from build123d import *

# Parameters (mm, degrees)
F1_DEPTH = 3
F2_W     = 3
F2_H     = 20
F3_DEPTH = 20
F4_R     = 3
F5_DEPTH = 3.001


with BuildPart() as f1:
    # F0 (on Top) → F1 (new body)
    with BuildSketch(Plane.XY):
        Polygon((0, 10), (0, 0), (0, -10), (35, -10), (35, 0), (35, 10), align=None)
        with BuildLine():
            ThreePointArc((29.466326, 0), (23.966326, -5.5), (18.466326, 0))
            ThreePointArc((18.466326, 0), (23.966326, 5.5), (29.466326, 0))
        make_face(mode=Mode.SUBTRACT)
    extrude(amount=F1_DEPTH)

    # F2 (on face) → F3 (join)
    with BuildSketch(Plane.XY.offset(3)):
        with Locations((1.5, 0)):
            Rectangle(F2_W, F2_H)
    extrude(amount=F3_DEPTH)

    # F4 (on face) → F5 (cut, through all)
    with BuildSketch(Plane.YZ.offset(3)):
        with Locations((0, 13)):
            Circle(F4_R)
    extrude(amount=-F5_DEPTH, mode=Mode.SUBTRACT)


solid = f1.part
Can you work these out from the model? Positions are in its coordinate system, mm. A direction names the side the tool comes from. Coordinates: 2 decimals unless noted, no trailing zeros. Loops run counter-clockwise (first coordinate to the right, second up) from the corner with the lowest first, then second, coordinate; pieces in that order, holes last. Notation, with made-up numbers: M -11,-34.5 L 1,-34.5 A18 ccw 1,-22.5 Z; hole C 40.25,15.25 d10. An arc over 180 degrees is marked long. Return JSON: item names as keys, results as strings. Group by question number.
Item 1: If I drill on L1, parallel to Z at x = 1.2, y = 0; L2, parallel to Z at x = 19, y = 5.75, over which ranges is the centre line in solid material (lowest first)? Write a range as from..to.
Item 2: Imagine slicing it at D-D (z = 13). Please give me the cut outline in (x, y).
Item 3: Imagine slicing it at C-C (x = 28). Please give me the cut outline in (y, z).
Item 4: Thinking about a two-plate mould opening in X: for faces 3 (the flat face through (0, 0, 9)), 4 (the cylindrical face through (28.02, 3.72, 1.48)), 5 (the flat face through (14, 10, 2)), which applies, released by +X, released by -X, zero draft, split by the parting line, or undercut?
Item 5: On a 3-axis mill with a long thin cutter (end or side, diameter ignored), from which of +Z, -Z, +X, -X, +Y, -Y can I reach the whole of each face in a straight line? I mean faces 1 (the flat face through (17, 0, 0)), 2 (the flat face through (18.8, 2.4, 3)). Say none if no direction works.
Item 6: Imagine slicing it at A-A (y = 0). Please give me the cut outline in (x, z).
Item 7: I'm going to push a flat-ended pin straight in: pin 1 Ø12 at (y, z) = (7, 14) entering from +X. Where does the tip first touch, or does it pass through?
Item 8: Imagine slicing it at B-B (z = 2.5). Please give me the cut outline in (x, y), and give its area (3 significant figures).
Verdict:
{
 "1": {"L1": "z = 0..10, 16..23", "L2": "z = 0..3"},
 "2": {"outline": "M 0,-10 L 3,-10 L 3,-3 L 0,-3 Z; M 0,3 L 3,3 L 3,10 L 0,10 Z"},
 "3": {"outline": "M -10,0 L -3.74,0 L -3.74,3 L -10,3 Z; M 3.74,0 L 10,0 L 10,3 L 3.74,3 Z"},
 "4": {"face 3": "released by -X", "face 4": "undercut", "face 5": "zero draft"},
 "5": {"face 1": "-Z, +X, -X, +Y, -Y", "face 2": "+Z, +X, +Y, -Y"},
 "6": {"outline": "M 0,0 L 18.47,0 L 18.47,3 L 3,3 L 3,10 L 0,10 Z; M 0,16 L 3,16 L 3,23 L 0,23 Z; M 29.47,0 L 35,0 L 35,3 L 29.47,3 Z"},
 "7": {"pin 1": "stops at x = 3"},
 "8": {"outline": "M 0,-10 L 35,-10 L 35,10 L 0,10 Z; hole C 23.97,0 d11", "area": "605 mm^2"}
}
